```python
from build123d import *

# Parameters (mm, degrees)
SKETCH_1_W          = 300
SKETCH_1_H          = 625
EXTRUDE_1_DEPTH     = 600
CUT_EXTRUDE_1_DEPTH = 600


with BuildPart() as part:
    # 草图1 → 凸台-拉伸1 (new body)
    with BuildSketch(Plane(origin=(0, 0, 0), x_dir=(1, 0, 0), z_dir=(0, 1, 0))):
        with Locations((150, 312.5)):
            Rectangle(SKETCH_1_W, SKETCH_1_H)
    extrude(amount=EXTRUDE_1_DEPTH)

    # 草图2 → 切除-拉伸1 (cut)
    with BuildSketch(Plane(origin=(300, 0, 0), x_dir=(0, 0, -1), z_dir=(1, 0, 0))):
        Polygon((365, 600), (0, 600), (0, 300), align=None)
    extrude(amount=-CUT_EXTRUDE_1_DEPTH, mode=Mode.SUBTRACT)


solid = part.part
```
Part model, mm, in its own coordinate system. Coordinates: 2 decimals unless noted, no trailing zeros. Write each loop counter-clockwise with the first axis right and the second up, starting at its lowest first coordinate (ties: lowest second). Pieces come first, ordered by that corner, then holes.
Item 1: Slice it at C-C (z = -54). Write the cut outline in (x, y), and give its area (3 significant figures).
Item 2: Probe line 1 (Y direction, x = 144, z = -336.5); line 2 (Z direction, x = 192, y = 329); line 3 (Y direction, x = 186, z = -93.5). List the from-to ranges inside material, lowest first.
Item 3: Pin check, flat tips, straight feed: pin 1 (6 mm diameter, centred on x = 189.5, y = 70, fed in from +Z); pin 2 (8 mm diameter, centred on x = 233, y = 395.5, fed in from +Z) (3 decimals); pin 3 (1.5 mm diameter, centred on x = 220.5, y = 463, fed in from +Z). Stop position of each tip, or through.
Item 4: Slice it at A-A (x = 224). Write the cut outline in (y, z).
Item 5: Slice it at B-B (y = 463). Write the cut outline in (x, z).
Results found:
1. outline: (0, 0) - (300, 0) - (300, 344.38) - (0, 344.38) - close
1. area: 103,000 mm2
2. line 1: y = 0 to 576.58
2. line 2: z = -625 to -35.28
2. line 3: y = 0 to 376.85
3. pin 1: stops at z = 0
3. pin 2: stops at z = -111.325
3. pin 3: stops at z = -197.4
4. outline: (0, -625) - (600, -625) - (600, -365) - (300, 0) - (0, 0) - close
5. outline: (0, -625) - (300, -625) - (300, -198.32) - (0, -198.32) - close
